from build123d import *

# Parameters (mm, degrees)
SKETCH2_W           = 50.8
SKETCH2_H           = 50.8
SKETCH2_W_2         = 44.45
SKETCH2_H_2         = 44.45
BOSS_EXTRUDE1_DEPTH = 127
SKETCH3_R           = 3.175
CUT_EXTRUDE1_DEPTH  = 140.121529606
SKETCH5_W           = 44.45
SKETCH5_H           = 44.45
CUT_EXTRUDE2_DEPTH  = 140.121529606
CHAMFER1_SIZE       = 12.7


with BuildPart() as part:
    # Sketch2 → Boss-Extrude1 (new body)
    with BuildSketch(Plane.XY):
        Rectangle(SKETCH2_W, SKETCH2_H)
        Rectangle(SKETCH2_W_2, SKETCH2_H_2, mode=Mode.SUBTRACT)
    extrude(amount=BOSS_EXTRUDE1_DEPTH)

    # Sketch3 → Cut-Extrude1 (cut, through all)
    with BuildSketch(Plane.ZY.offset(25.4)):
        with Locations((25.4, 0)):
            Circle(SKETCH3_R)
    extrude(amount=-CUT_EXTRUDE1_DEPTH, mode=Mode.SUBTRACT)

    # Sketch5 → Cut-Extrude2 (cut, through all)
    with BuildSketch(Plane(origin=(0, 25.4, 0), x_dir=(1, 0, 0), z_dir=(0, 1, 0))):
        with Locations((0, -22.225)):
            Rectangle(SKETCH5_W, SKETCH5_H)
    extrude(amount=-CUT_EXTRUDE2_DEPTH, mode=Mode.SUBTRACT)

    # Chamfer1
    chamfer1_edges = [part.edges().sort_by_distance(p)[0] for p in [
        (23.8125, -25.4, 0),
        (-23.8125, 25.4, 0),
        (-23.8125, -25.4, 0),
        (23.8125, 25.4, 0),
    ]]
    chamfer(chamfer1_edges, length=CHAMFER1_SIZE)


solid = part.part
Build history of the part. All positions in model axes, mm. A direction names the side the tool comes from. Give positions to 0.01 mm unless a question says otherwise; leave off trailing zeros. Loops run counter-clockwise (first coordinate to the right, second up) from the corner with the lowest first, then second, coordinate; pieces in that order, holes last. Notation, with made-up numbers: (69, 33) -> (113, 33) arc R18 ccw to (113, 39) -> close; hole circle Ø8 at (78.25, 27). An arc over 180 degrees is marked (long way). Answer in a Markdown table with one row per item.
Item 1: Flat gauge pins, fed straight in: P1, Ø8.5, axis at y = 0, z = 25.4, coming from the +X side; P2, Ø1.6, axis at x = 8.5, y = -24, coming from the -Z side; P3, Ø5, axis at x = 19, y = -2, coming from the -Z side. Where does each tip first touch, or does it go through?
Findings below:
| item | result |
|---|---|
| P1 | stops at x = 25.4 |
| P2 | stops at z = 44.45 |
| P3 | passes through |
Item 2: Slice it at C-C on y = 17.5. Write the cut outline in (x, z) (3 decimals).
Findings below:
| item | result |
|---|---|
| outline | (-25.4, 4.8) -> (-22.225, 4.8) -> (-22.225, 127) -> (-25.4, 127) -> close; (22.225, 4.8) -> (25.4, 4.8) -> (25.4, 127) -> (22.225, 127) -> close |
Item 3: Probe line 1 along X through (y, z) = (16, 34) (3 decimals); line 2 along Y through (x, z) = (-23, 25). List the from-to ranges inside material, lowest first. Write a range as [from, to].
Findings below:
| item | result |
|---|---|
| line 1 | x = [-25.4, -22.225], [22.225, 25.4] |
| line 2 | y = [-25.4, -3.15], [3.15, 25.4] |
Item 4: Slice it at D-D on x = 18.5. Write the cut outline in (y, z) (3 decimals), plus the area to 3 significant figures.
Findings below:
| item | result |
|---|---|
| outline | (-25.4, 44.45) -> (-22.225, 44.45) -> (-22.225, 127) -> (-25.4, 127) -> close; (22.225, 44.45) -> (25.4, 44.45) -> (25.4, 127) -> (22.225, 127) -> close |
| area | 524 mm² |
Item 5: Tool access for faces 1 (the flat face through (0, -24, 44.45)), 2 (the flat face through (0, -22.225, 85)), 3 (the flat face through (23.8, 19.1, 6.4)): list every direction of +Z, -Z, +X, -X, +Y, -Y with a clear straight run to the whole face (end or side of a thin tool).
Findings below:
| item | result |
|---|---|
| face 1 | -Z, +Y, -Y |
| face 2 | +Z, -Z |
| face 3 | -Z, +X, -X, +Y |
Item 6: Slice it at B-B on y = 0. Write the cut outline in (x, z) (3 decimals).
Findings below:
| item | result |
|---|---|
| outline | (-25.4, 0) -> (-22.225, 0) -> (-22.225, 22.225) -> (-25.4, 22.225) -> close; (-25.4, 28.575) -> (-22.225, 28.575) -> (-22.225, 127) -> (-25.4, 127) -> close; (22.225, 0) -> (25.4, 0) -> (25.4, 22.225) -> (22.225, 22.225) -> close; (22.225, 28.575) -> (25.4, 28.575) -> (25.4, 127) -> (22.225, 127) -> close |
Item 7: Slice it at A-A on z = 50.5. Write the cut outline in (x, y) (3 decimals), plus the area to 3 significant figures.
Findings below:
| item | result |
|---|---|
| outline | (-25.4, -25.4) -> (25.4, -25.4) -> (25.4, 25.4) -> (-25.4, 25.4) -> close; hole (-22.225, -22.225) -> (22.225, -22.225) -> (22.225, 22.225) -> (-22.225, 22.225) -> close |
| area | 605 mm² |
Item 8: Mould opens along Z. For faces 4 (the flat face through (-23, 0, 127)), 5 (the cylindrical face through (-23.83, 0.95, 28.43)), 6 (the flat face through (0, -25.4, 82)), 7 (the flat face through (24, 0, 0)) say: pulls with the +Z half, pulls with the -Z half, needs draft (parallel to the pull), parting line crosses it, or undercut.
Findings below:
| item | result |
|---|---|
| face 4 | pulls with the +Z half |
| face 5 | undercut |
| face 6 | needs draft |
| face 7 | pulls with the -Z half |
